from build123d import *

# Parameters (mm, degrees)
SKETCH1_W           = 193
SKETCH1_H           = 145
SKETCH1_W_2         = 35
SKETCH1_H_2         = 60
BOSS_EXTRUDE1_DEPTH = 1
SKETCH2_R           = 2.5
CUT_EXTRUDE1_DEPTH  = 3
SKETCH3_W           = 1.5
SKETCH3_H           = 60.155824732
SKETCH3_H_2         = 60
CUT_EXTRUDE2_DEPTH  = 3
SKETCH4_W           = 193
SKETCH4_H           = 42
BOSS_EXTRUDE2_DEPTH = 1
SKETCH5_W           = 1
SKETCH5_H           = 25
BOSS_EXTRUDE3_DEPTH = 194
CHAMFER1_SIZE       = 2
SKETCH7_W           = 36.5
SKETCH7_H           = 3
CUT_EXTRUDE3_DEPTH  = 10
SKETCH8_R           = 2.5
CUT_EXTRUDE4_DEPTH  = 10
SKETCH11_W          = 1
SKETCH11_H          = 25
CUT_EXTRUDE5_DEPTH  = 1
CUT_EXTRUDE6_DEPTH  = 10


with BuildPart() as part:
    # Sketch1 → Boss-Extrude1 (new body)
    with BuildSketch(Plane.XY):
        Rectangle(SKETCH1_W, SKETCH1_H)
        with Locations((-77.5, 35.5)):
            Rectangle(SKETCH1_W_2, SKETCH1_H_2, mode=Mode.SUBTRACT)
        with Locations((77.5, 35.5)):
            Rectangle(SKETCH1_W_2, SKETCH1_H_2, mode=Mode.SUBTRACT)
        with Locations((77.5, -39.5)):
            Rectangle(SKETCH1_W_2, SKETCH1_H_2, mode=Mode.SUBTRACT)
        with Locations((-77.5, -39.5)):
            Rectangle(SKETCH1_W_2, SKETCH1_H_2, mode=Mode.SUBTRACT)
    extrude(amount=BOSS_EXTRUDE1_DEPTH)

    # Sketch2 → Cut-Extrude1 (cut)
    with BuildSketch(Plane.XY.offset(1)):
        with Locations((-53, 45.5)):
            Circle(SKETCH2_R)
        with Locations((-53, 25.5)):
            Circle(SKETCH2_R)
        with Locations((-53, -49.5)):
            Circle(SKETCH2_R)
        with Locations((-53, -29.5)):
            Circle(SKETCH2_R)
        with Locations((53, -29.5)):
            Circle(SKETCH2_R)
        with Locations((53, -49.5)):
            Circle(SKETCH2_R)
        with Locations((53, 25.5)):
            Circle(SKETCH2_R)
        with Locations((53, 45.5)):
            Circle(SKETCH2_R)
    extrude(amount=-CUT_EXTRUDE1_DEPTH, mode=Mode.SUBTRACT)

    # Sketch3 → Cut-Extrude2 (cut)
    with BuildSketch(Plane.XY.offset(1)):
        with Locations((-95.75, 35.422087634)):
            Rectangle(SKETCH3_W, SKETCH3_H)
        with Locations((-95.75, -39.5)):
            Rectangle(SKETCH3_W, SKETCH3_H_2)
        with Locations((95.75, -39.5)):
            Rectangle(SKETCH3_W, SKETCH3_H_2)
        with Locations((95.75, 35.5)):
            Rectangle(SKETCH3_W, SKETCH3_H_2)
    extrude(amount=-CUT_EXTRUDE2_DEPTH, mode=Mode.SUBTRACT)

    # Sketch4 → Boss-Extrude2 (add)
    with BuildSketch(Plane.XY.offset(1)):
        with Locations((0, 93.5)):
            Rectangle(SKETCH4_W, SKETCH4_H)
    extrude(amount=-BOSS_EXTRUDE2_DEPTH)

    # Sketch5 → Boss-Extrude3 (add)
    with BuildSketch(Plane.ZY.offset(96.5)):
        with Locations((0.5, -2.240916736)):
            Rectangle(SKETCH5_W, SKETCH5_H)
    extrude(amount=-BOSS_EXTRUDE3_DEPTH)

    # Chamfer1
    # the kernel refuses this chamfer: 2 mm, written as the material it takes off along each edge
    with BuildSketch(Plane(origin=(101.643365976, 114.5, 1), x_dir=(0, -0.9996219169112968, 0.027495876610586306), z_dir=(-1, 0, 0))) as chamfer1_piece_1:
        Polygon((CHAMFER1_SIZE * 0.999621916911, -CHAMFER1_SIZE * 0.0274958766106), (-CHAMFER1_SIZE * 0.0274958766106, -CHAMFER1_SIZE * 0.999621916911), (0, 0), align=None)
    extrude(amount=203.286731952, mode=Mode.SUBTRACT)

    # Sketch7 → Cut-Extrude3 (cut)
    with BuildSketch(Plane.XY.offset(1)):
        with Locations((-78.25, -71)):
            Rectangle(SKETCH7_W, SKETCH7_H)
        with Locations((78.25, -71)):
            Rectangle(SKETCH7_W, SKETCH7_H)
    extrude(amount=-CUT_EXTRUDE3_DEPTH, mode=Mode.SUBTRACT)

    # Sketch8 → Cut-Extrude4 (cut)
    with BuildSketch(Plane.XY.offset(1)):
        with Locations((-22, 45.5)):
            Circle(SKETCH8_R)
        with Locations((-22, 25.5)):
            Circle(SKETCH8_R)
        with Locations((22, -29.5)):
            Circle(SKETCH8_R)
        with Locations((22, -49.5)):
            Circle(SKETCH8_R)
    extrude(amount=-CUT_EXTRUDE4_DEPTH, mode=Mode.SUBTRACT)

    # Sketch11 → Cut-Extrude5 (cut)
    with BuildSketch(Plane(origin=(97.5, 0, 0), x_dir=(0, 0, -1), z_dir=(1, 0, 0))):
        with Locations((-0.5, -2.240916736)):
            Rectangle(SKETCH11_W, SKETCH11_H)
    extrude(amount=-CUT_EXTRUDE5_DEPTH, mode=Mode.SUBTRACT)

    # Sketch12 → Cut-Extrude6 (cut)
    with BuildSketch(Plane.XY.offset(1)):
        with BuildLine():
            Line((-50.5, 48), (-50.5, 43))
            ThreePointArc((-50.5, 43), (-53, 40.5), (-55.5, 43))
            Line((-55.5, 43), (-55.5, 48))
            ThreePointArc((-55.5, 48), (-53, 50.5), (-50.5, 48))
        make_face()
        with BuildLine():
            Line((-19.5, 48), (-19.5, 43))
            ThreePointArc((-19.5, 43), (-22, 40.5), (-24.5, 43))
            Line((-24.5, 43), (-24.5, 48))
            ThreePointArc((-24.5, 48), (-22, 50.5), (-19.5, 48))
        make_face()
        with BuildLine():
            Line((-19.5, 28), (-19.5, 23))
            ThreePointArc((-19.5, 23), (-22, 20.5), (-24.5, 23))
            Line((-24.5, 23), (-24.5, 28))
            ThreePointArc((-24.5, 28), (-22, 30.5), (-19.5, 28))
        make_face()
        with BuildLine():
            Line((-50.5, 28), (-50.5, 23))
            ThreePointArc((-50.5, 23), (-53, 20.5), (-55.5, 23))
            Line((-55.5, 23), (-55.5, 28))
            ThreePointArc((-55.5, 28), (-53, 30.5), (-50.5, 28))
        make_face()
        with BuildLine():
            Line((50.5, 28), (50.5, 23))
            ThreePointArc((50.5, 23), (53, 20.5), (55.5, 23))
            Line((55.5, 23), (55.5, 28))
            ThreePointArc((55.5, 28), (53, 30.5), (50.5, 28))
        make_face()
        with BuildLine():
            Line((50.5, 48), (50.5, 43))
            ThreePointArc((50.5, 43), (53, 40.5), (55.5, 43))
            Line((55.5, 43), (55.5, 48))
            ThreePointArc((55.5, 48), (53, 50.5), (50.5, 48))
        make_face()
        with BuildLine():
            Line((50.5, -52.481833472), (50.5, -47.481833472))
            ThreePointArc((50.5, -47.481833472), (53, -44.981833472), (55.5, -47.481833472))
            Line((55.5, -47.481833472), (55.5, -52.481833472))
            ThreePointArc((55.5, -52.481833472), (53, -54.981833472), (50.5, -52.481833472))
        make_face()
        with BuildLine():
            Line((50.5, -32.481833472), (50.5, -27.481833472))
            ThreePointArc((50.5, -27.481833472), (53, -24.981833472), (55.5, -27.481833472))
            Line((55.5, -27.481833472), (55.5, -32.481833472))
            ThreePointArc((55.5, -32.481833472), (53, -34.981833472), (50.5, -32.481833472))
        make_face()
        with BuildLine():
            Line((-50.5, -32.481833472), (-50.5, -27.481833472))
            ThreePointArc((-50.5, -27.481833472), (-53, -24.981833472), (-55.5, -27.481833472))
            Line((-55.5, -27.481833472), (-55.5, -32.481833472))
            ThreePointArc((-55.5, -32.481833472), (-53, -34.981833472), (-50.5, -32.481833472))
        make_face()
        with BuildLine():
            Line((-50.5, -52.481833472), (-50.5, -47.481833472))
            ThreePointArc((-50.5, -47.481833472), (-53, -44.981833472), (-55.5, -47.481833472))
            Line((-55.5, -47.481833472), (-55.5, -52.481833472))
            ThreePointArc((-55.5, -52.481833472), (-53, -54.981833472), (-50.5, -52.481833472))
        make_face()
        with BuildLine():
            Line((24.5, -27), (24.5, -32))
            ThreePointArc((24.5, -32), (22, -34.5), (19.5, -32))
            Line((19.5, -32), (19.5, -27))
            ThreePointArc((19.5, -27), (22, -24.5), (24.5, -27))
        make_face()
        with BuildLine():
            Line((24.5, -47), (24.5, -52))
            ThreePointArc((24.5, -52), (22, -54.5), (19.5, -52))
            Line((19.5, -52), (19.5, -47))
            ThreePointArc((19.5, -47), (22, -44.5), (24.5, -47))
        make_face()
    extrude(amount=-CUT_EXTRUDE6_DEPTH, mode=Mode.SUBTRACT)


solid = part.part
Geometry: final body of the model. Coordinates: model frame, mm. Round coordinates to 2 decimals unless told otherwise and drop trailing zeros. Loops run counter-clockwise (first coordinate to the right, second up) from the corner with the lowest first, then second, coordinate; pieces in that order, holes last. Notation, with made-up numbers: M -40,-31.5 L -32,-31.5 A7 cw -32,-22.5 Z; hole C 15.25,23.25 d8. An arc over 180 degrees is marked long. Put each result on its own line as item: value. Start each with the question number.
(1) Section query B-B (x = -79). Return loops of the section in (y, z), then the cut area to 3 significant figures.
(2) Section query A-A (x = 22). Return loops of the section in (y, z), then the cut area to 4 significant figures.
(3) Section query C-C (x = 53). Return loops of the section in (y, z), then the cut area to 4 significant figures.
(4) Material intervals for line 1 along Y through (x, z) = (54, 0.85); line 2 along X through (y, z) = (-26.5, 0.3); line 3 along X through (y, z) = (41, 0.2), sorted ascending. Write a range as [from, to].
(5) Section query D-D (z = 0.6). State how many separate pieces and enclosed holes the cut face has, then the cut area to 3 significant figures.
(6) Contact query for flat-ended pins moving along their axis: pin 1 Ø0.5 at (y, z) = (25.5, 0.5) entering from -X; pin 2 Ø0.5 at (y, z) = (-49.5, 0.5) entering from +X. Output: stop coordinate, or through.
Findings below:
1. outline: M -14.74,0 L 10.26,0 L 10.26,1 L -14.74,1 Z; M 65.5,0 L 113.5,0 L 112.5,1 L 65.5,1 Z
1. area: 72.5 mm2
2. outline: M -72.5,0 L -54.5,0 L -54.5,1 L -72.5,1 Z; M -44.5,0 L -34.5,0 L -34.5,1 L -44.5,1 Z; M -24.5,0 L 113.5,0 L 112.5,1 L -24.5,1 Z
2. area: 165.5 mm2
3. outline: M -72.5,0 L -54.98,0 L -54.98,1 L -72.5,1 Z; M -44.98,0 L -34.98,0 L -34.98,1 L -44.98,1 Z; M -24.98,0 L 20.5,0 L 20.5,1 L -24.98,1 Z; M 30.5,0 L 40.5,0 L 40.5,1 L 30.5,1 Z; M 50.5,0 L 113.5,0 L 112.5,1 L 50.5,1 Z
3. area: 145.5 mm2
4. line 1: y = [-72.5, -54.77], [-45.19, -34.77], [-25.19, 20.71], [30.29, 40.71], [50.29, 112.65]
4. line 2: x = [-60, -55.3], [-50.7, 19.55], [24.45, 50.7], [55.3, 60]
4. line 3: x = [-60, -54.5], [-51.5, -23.5], [-20.5, 51.5], [54.5, 60]
5. separate pieces: 1
5. enclosed holes: 12
5. area: 27,000 mm2
6. pin 1: stops at x = -60
6. pin 2: stops at x = 60
